from build123d import *

# Parameters (mm, degrees)
CYLINDER006_R                 = 1.5
CYLINDER006_DEPTH             = 12
LINEAREXTRUDE004_DEPTH        = 10
DIFFERENCE005_PLACEMENT_ANGLE = -10


with BuildPart() as cylinder006:
    # cylinder006 → cylinder006 (new body)
    with BuildSketch(Plane.XY.offset(-1)):
        Circle(CYLINDER006_R)
    extrude(amount=CYLINDER006_DEPTH)


with BuildPart() as difference005:
    # union006 → LinearExtrude004 (new body)
    with BuildSketch(Plane(origin=(0, 0, 0), x_dir=(0, 1, 0), z_dir=(0, 0, 1))):
        Polygon((0.711931, -4.306123), (1.370771, -4.143733), (1.502069, -4.540636), (1.530367, -4.602072), (1.641751, -4.771632), (1.871155, -5.020002), (2.245545, -5.309618), (2.782207, -5.596589), (3.025427, -5.468937), (3.094113, -4.864255), (3.068442, -4.391617), (2.994354, -4.061731), (2.918082, -3.873743), (2.883597, -3.815555), (2.631538, -3.482032), (3.139447, -3.032064), (3.440155, -3.322487), (3.493763, -3.363735), (3.671187, -3.46211), (3.989737, -3.575421), (4.455834, -3.657875), (5.064387, -3.662577), (5.220426, -3.436516), (5.000234, -2.869177), (4.757857, -2.462607), (4.53895, -2.204938), (4.384052, -2.073928), (4.326475, -2.038431), (3.948292, -1.860249), (4.188912, -1.225786), (4.590143, -1.343197), (4.656779, -1.354807), (4.859597, -1.359461), (5.194318, -1.311756), (5.645345, -1.168159), (6.186377, -0.889514), (6.219486, -0.616832), (5.76086, -0.216806), (5.357304, 0.030555), (5.043726, 0.156979), (4.845688, 0.200998), (4.77821, 0.205671), (4.36054, 0.187693), (4.278749, 0.861305), (4.688584, 0.943805), (4.752983, 0.964491), (4.934732, 1.054624), (5.208943, 1.252418), (5.541575, 1.58917), (5.891142, 2.087328), (5.793738, 2.344162), (5.201743, 2.485233), (4.729457, 2.516719), (4.393046, 2.482935), (4.197235, 2.429879), (4.135314, 2.402658), (3.773841, 2.192639), (3.388376, 2.751081), (3.712928, 3.01459), (3.760337, 3.062835), (3.879381, 3.227107), (4.030263, 3.529677), (4.168298, 3.982437), (4.246318, 4.585986), (4.040715, 4.768136), (3.45097, 4.617935), (3.018149, 4.426332), (2.735972, 4.240079), (2.587247, 4.102103), (2.545069, 4.049224), (2.322601, 3.695276), (1.721767, 4.010618), (1.886685, 4.394771), (1.906243, 4.459522), (1.93531, 4.6603), (1.928298, 4.99833), (1.840114, 5.463378), (1.628715, 6.034052), (1.362012, 6.099788), (0.909622, 5.692724), (0.61542, 5.321926), (0.452121, 5.025874), (0.384552, 4.834585), (0.371779, 4.768162), (0.339281, 4.351371), (-0.339281, 4.351371), (-0.371779, 4.768162), (-0.384552, 4.834585), (-0.452121, 5.025874), (-0.61542, 5.321926), (-0.909622, 5.692724), (-1.362012, 6.099788), (-1.628715, 6.034052), (-1.840114, 5.463378), (-1.928298, 4.99833), (-1.93531, 4.6603), (-1.906243, 4.459522), (-1.886685, 4.394771), (-1.721767, 4.010618), (-2.322601, 3.695276), (-2.545069, 4.049224), (-2.587247, 4.102103), (-2.735972, 4.240079), (-3.018149, 4.426332), (-3.45097, 4.617935), (-4.040715, 4.768136), (-4.246318, 4.585986), (-4.168298, 3.982437), (-4.030263, 3.529677), (-3.879381, 3.227107), (-3.760337, 3.062835), (-3.712928, 3.01459), (-3.388376, 2.751081), (-3.773841, 2.192638), (-4.135314, 2.402658), (-4.197235, 2.429879), (-4.393046, 2.482935), (-4.729457, 2.516719), (-5.201743, 2.485233), (-5.793738, 2.344162), (-5.891142, 2.087328), (-5.541575, 1.58917), (-5.208943, 1.252418), (-4.934732, 1.054624), (-4.752983, 0.964491), (-4.688584, 0.943805), (-4.278749, 0.861305), (-4.36054, 0.187693), (-4.77821, 0.205671), (-4.845688, 0.200998), (-5.043726, 0.156979), (-5.357304, 0.030555), (-5.76086, -0.216806), (-6.219486, -0.616832), (-6.186377, -0.889514), (-5.645345, -1.168159), (-5.194318, -1.311756), (-4.859597, -1.359461), (-4.656779, -1.354807), (-4.590143, -1.343197), (-4.188912, -1.225786), (-3.948292, -1.860249), (-4.326475, -2.038431), (-4.384052, -2.073928), (-4.53895, -2.204938), (-4.757857, -2.462607), (-5.000234, -2.869177), (-5.220426, -3.436516), (-5.064387, -3.662577), (-4.455834, -3.657875), (-3.989737, -3.575421), (-3.671187, -3.46211), (-3.493763, -3.363735), (-3.440155, -3.322487), (-3.139447, -3.032064), (-2.631537, -3.482032), (-2.883597, -3.815555), (-2.918082, -3.873743), (-2.994354, -4.061731), (-3.068442, -4.391617), (-3.094113, -4.864255), (-3.025427, -5.468937), (-2.782207, -5.596589), (-2.245545, -5.309618), (-1.871155, -5.020002), (-1.641751, -4.771632), (-1.530367, -4.602072), (-1.502069, -4.540636), (-1.370771, -4.143733), (-0.71193, -4.306122), (-0.780122, -4.71858), (-0.783616, -4.78613), (-0.763789, -4.98803), (-0.676085, -5.31456), (-0.47917, -5.74499), (-0.137342, -6.24849), (0.137342, -6.24849), (0.47917, -5.74499), (0.676085, -5.31456), (0.763789, -4.98803), (0.783616, -4.78613), (0.780122, -4.71858), align=None)
    extrude(amount=LINEAREXTRUDE004_DEPTH)

    # difference005: cut cylinder006
    add(cylinder006.part, mode=Mode.SUBTRACT)


with BuildPart() as difference005_1:
    # difference005 placement: moved
    add(difference005.part.moved(Location((-5.5, 9.53, 0))).rotate(Axis((-5.5, 9.53, 0), (0, 0, 1)), DIFFERENCE005_PLACEMENT_ANGLE))


solid = difference005_1.part
Design review of the part built by this model. Coordinates are the model's own, in mm. Round coordinates to 2 decimals unless told otherwise and drop trailing zeros. Answer as CSV lines item,"result". Start each with the question number.
1) For pin 1 Ø5 at (x, z) = (-7, 1) entering from +Y; pin 2 Ø3 at (y, z) = (13, 7) entering from +X; pin 3 Ø3 at (x, z) = (-10.5, 3) entering from -Y; pin 4 Ø2.5 at (x, y) = (-5.5, 9.53) entering from -Z, all flat-tipped, find the tip position at first contact; note any pin that passes through.
2) The part is to be moulded in two halves that separate along Y. For faces 1 (the face through (-6.075, 8.144, 4.93)), 2 (the face through (-4, 11, 0)), say which applies: +Y half, -Y half, draft (parallel to the pull), parting line (faces both ways), or undercut.
3) Wall thickness on line 1 along Y through (x, z) = (-1.5, 0.75); line 2 along Y through (x, z) = (-10, 1.5); line 3 along X through (y, z) = (13.75, 2.25): over which ranges is each line inside the solid? List them lowest first. Write a range as [from, to].
Resolved:
1,pin 1,"y = 15.69"
1,pin 2,"x = 0.43"
1,pin 3,"y = 6.12"
1,pin 4,"through"
2,face 1,"undercut"
2,face 2,"draft"
3,line 1,"[5.7, 7.38], [7.82, 11.58], [12.49, 14.02]"
3,line 2,"[6.13, 7.69], [8.47, 9.97], [10.69, 12.28]"
3,line 3,"[-9.45, -7.85], [-7.05, -3.41], [-2.31, -1.04]"
